```python
from build123d import *

# Parameters (mm, degrees)
F1_DEPTH     = 2
F2_W         = 44.2697719236
F2_H         = 2
F2_W_2       = 43.7677401211
F2_W_3       = 43.2657083186
F2_W_4       = 42.7408568887
F2_W_5       = 42.1931858314
F2_W_6       = 41.5998755193
F2_W_7       = 40.9609259524
F2_W_8       = 40.2763371308
F2_W_9       = 39.5461090544
F2_W_10      = 38.7702417233
F2_W_11      = 37.9487351373
F2_W_12      = 37.0815892966
F2_W_13      = 36.1688042011
F2_W_14      = 35.2103798508
F2_W_15      = 34.2063162458
F3_DEPTH     = 1
F4_T1_DEPTH  = 50.2158074986
F4_T3_DEPTH  = 3.0186569416
F4_T5_DEPTH  = 47.197150557
F4_T7_DEPTH  = 49.7137756961
F4_T9_DEPTH  = 49.2117438936
F4_T11_DEPTH = 48.6868924637
F4_T13_DEPTH = 48.1392214064
F4_T15_DEPTH = 47.5459110943
F4_T17_DEPTH = 46.9069615275
F4_T19_DEPTH = 46.2223727058
F4_T21_DEPTH = 45.4921446294
F4_T23_DEPTH = 44.7162772983
F4_T25_DEPTH = 43.8947707123
F4_T27_DEPTH = 43.0276248716
F4_T29_DEPTH = 42.1148397761
F4_T31_DEPTH = 41.1564154259
F4_T33_DEPTH = 40.1523518208


# Not quite as in the source:
# - a fillet or chamfer that OpenCascade refuses, or shapes differently, is made with other operations: its cross-section is extruded or revolved along the edge and cut away or added


with BuildPart() as f1:
    # F0 (on Top) → F1 (new body)
    with BuildSketch(Plane.XY):
        Polygon((17.9405650105, 218.366242675), (-15.0594349895, 218.366242675), (-21.0594349895, -44.5653073527), (23.9405650105, -44.5653073527), align=None)
    extrude(amount=F1_DEPTH)

    # F2 (on face) → F3 (join)
    with BuildSketch(Plane.XY.offset(2)):
        with Locations((1.4633846378, -28.5653073527)):
            Rectangle(F2_W, F2_H)
        with Locations((1.4405650105, -18.5653073527)):
            Rectangle(F2_W_2, F2_H)
        with Locations((1.4405650105, -7.5653073527)):
            Rectangle(F2_W_3, F2_H)
        with Locations((1.4405650105, 3.9346926473)):
            Rectangle(F2_W_4, F2_H)
        with Locations((1.4405650105, 15.9346926473)):
            Rectangle(F2_W_5, F2_H)
        with Locations((1.4405650105, 28.9346926473)):
            Rectangle(F2_W_6, F2_H)
        with Locations((1.4405650105, 42.9346926473)):
            Rectangle(F2_W_7, F2_H)
        with Locations((1.4405650105, 57.9346926473)):
            Rectangle(F2_W_8, F2_H)
        with Locations((1.4405650105, 73.9346926473)):
            Rectangle(F2_W_9, F2_H)
        with Locations((1.4405650105, 90.9346926473)):
            Rectangle(F2_W_10, F2_H)
        with Locations((1.4405650105, 108.9346926473)):
            Rectangle(F2_W_11, F2_H)
        with Locations((1.4405650105, 127.9346926473)):
            Rectangle(F2_W_12, F2_H)
        with Locations((1.4405650105, 147.9346926473)):
            Rectangle(F2_W_13, F2_H)
        with Locations((1.4405650105, 168.9346926473)):
            Rectangle(F2_W_14, F2_H)
        with Locations((1.4405650105, 190.9346926473)):
            Rectangle(F2_W_15, F2_H)
    extrude(amount=F3_DEPTH)

    # F4: fillet of radius 1.2071067812 on 30 edges, made by hand

    # F4_s2 → F4_t1 (cut)
    with BuildSketch(Plane.YZ.offset(-23.6445191115)):
        with BuildLine():
            ThreePointArc((-29.5653073527, 2), (-29.1529872247, 2.7167727513), (-28.3761002377, 3))
            Line((-28.3761002377, 3), (-29.5653073527, 3))
            Line((-29.5653073527, 3), (-29.5653073527, 2))
        make_face()
    extrude(amount=F4_T1_DEPTH, mode=Mode.SUBTRACT)

    # F4_s4 → F4_t3 (cut)
    with BuildSketch(Plane.YZ.offset(23.5526314455)):
        with BuildLine():
            ThreePointArc((-27.5653073527, 2), (-27.9776274807, 2.7167727513), (-28.7545144677, 3))
            Line((-28.7545144677, 3), (-27.5653073527, 3))
            Line((-27.5653073527, 3), (-27.5653073527, 2))
        make_face()
    extrude(amount=F4_T3_DEPTH, mode=Mode.SUBTRACT)

    # F4_s6 → F4_t5 (cut)
    with BuildSketch(Plane.YZ.offset(-23.6445191115)):
        with BuildLine():
            ThreePointArc((-27.5653073527, 2), (-27.9776274807, 2.7167727513), (-28.7545144677, 3))
            Line((-28.7545144677, 3), (-27.5653073527, 3))
            Line((-27.5653073527, 3), (-27.5653073527, 2))
        make_face()
    extrude(amount=F4_T5_DEPTH, mode=Mode.SUBTRACT)

    # F4_s8 → F4_t7 (cut)
    with BuildSketch(Plane.YZ.offset(-23.4163228376)):
        with BuildLine():
            ThreePointArc((-19.5653073527, 2), (-19.1529872247, 2.7167727513), (-18.3761002377, 3))
            Line((-18.3761002377, 3), (-19.5653073527, 3))
            Line((-19.5653073527, 3), (-19.5653073527, 2))
        make_face()
        with BuildLine():
            ThreePointArc((-17.5653073527, 2), (-17.9776274807, 2.7167727513), (-18.7545144677, 3))
            Line((-18.7545144677, 3), (-17.5653073527, 3))
            Line((-17.5653073527, 3), (-17.5653073527, 2))
        make_face()
    extrude(amount=F4_T7_DEPTH, mode=Mode.SUBTRACT)

    # F4_s10 → F4_t9 (cut)
    with BuildSketch(Plane.YZ.offset(-23.1653069363)):
        with BuildLine():
            ThreePointArc((-8.5653073527, 2), (-8.1529872247, 2.7167727513), (-7.3761002377, 3))
            Line((-7.3761002377, 3), (-8.5653073527, 3))
            Line((-8.5653073527, 3), (-8.5653073527, 2))
        make_face()
        with BuildLine():
            ThreePointArc((-6.5653073527, 2), (-6.9776274807, 2.7167727513), (-7.7545144677, 3))
            Line((-7.7545144677, 3), (-6.5653073527, 3))
            Line((-6.5653073527, 3), (-6.5653073527, 2))
        make_face()
    extrude(amount=F4_T9_DEPTH, mode=Mode.SUBTRACT)

    # F4_s12 → F4_t11 (cut)
    with BuildSketch(Plane.YZ.offset(-22.9028812214)):
        with BuildLine():
            ThreePointArc((2.9346926473, 2), (3.3470127753, 2.7167727513), (4.1238997623, 3))
            Line((4.1238997623, 3), (2.9346926473, 3))
            Line((2.9346926473, 3), (2.9346926473, 2))
        make_face()
        with BuildLine():
            ThreePointArc((4.9346926473, 2), (4.5223725193, 2.7167727513), (3.7454855323, 3))
            Line((3.7454855323, 3), (4.9346926473, 3))
            Line((4.9346926473, 3), (4.9346926473, 2))
        make_face()
    extrude(amount=F4_T11_DEPTH, mode=Mode.SUBTRACT)

    # F4_s14 → F4_t13 (cut)
    with BuildSketch(Plane.YZ.offset(-22.6290456927)):
        with BuildLine():
            ThreePointArc((14.9346926473, 2), (15.3470127753, 2.7167727513), (16.1238997623, 3))
            Line((16.1238997623, 3), (14.9346926473, 3))
            Line((14.9346926473, 3), (14.9346926473, 2))
        make_face()
        with BuildLine():
            ThreePointArc((16.9346926473, 2), (16.5223725193, 2.7167727513), (15.7454855323, 3))
            Line((15.7454855323, 3), (16.9346926473, 3))
            Line((16.9346926473, 3), (16.9346926473, 2))
        make_face()
    extrude(amount=F4_T13_DEPTH, mode=Mode.SUBTRACT)

    # F4_s16 → F4_t15 (cut)
    with BuildSketch(Plane.YZ.offset(-22.3323905367)):
        with BuildLine():
            ThreePointArc((27.9346926473, 2), (28.3470127753, 2.7167727513), (29.1238997623, 3))
            Line((29.1238997623, 3), (27.9346926473, 3))
            Line((27.9346926473, 3), (27.9346926473, 2))
        make_face()
        with BuildLine():
            ThreePointArc((29.9346926473, 2), (29.5223725193, 2.7167727513), (28.7454855323, 3))
            Line((28.7454855323, 3), (29.9346926473, 3))
            Line((29.9346926473, 3), (29.9346926473, 2))
        make_face()
    extrude(amount=F4_T15_DEPTH, mode=Mode.SUBTRACT)

    # F4_s18 → F4_t17 (cut)
    with BuildSketch(Plane.YZ.offset(-22.0129157533)):
        with BuildLine():
            ThreePointArc((41.9346926473, 2), (42.3470127753, 2.7167727513), (43.1238997623, 3))
            Line((43.1238997623, 3), (41.9346926473, 3))
            Line((41.9346926473, 3), (41.9346926473, 2))
        make_face()
        with BuildLine():
            ThreePointArc((43.9346926473, 2), (43.5223725193, 2.7167727513), (42.7454855323, 3))
            Line((42.7454855323, 3), (43.9346926473, 3))
            Line((43.9346926473, 3), (43.9346926473, 2))
        make_face()
    extrude(amount=F4_T17_DEPTH, mode=Mode.SUBTRACT)

    # F4_s20 → F4_t19 (cut)
    with BuildSketch(Plane.YZ.offset(-21.6706213425)):
        with BuildLine():
            ThreePointArc((56.9346926473, 2), (57.3470127753, 2.7167727513), (58.1238997623, 3))
            Line((58.1238997623, 3), (56.9346926473, 3))
            Line((56.9346926473, 3), (56.9346926473, 2))
        make_face()
        with BuildLine():
            ThreePointArc((58.9346926473, 2), (58.5223725193, 2.7167727513), (57.7454855323, 3))
            Line((57.7454855323, 3), (58.9346926473, 3))
            Line((58.9346926473, 3), (58.9346926473, 2))
        make_face()
    extrude(amount=F4_T19_DEPTH, mode=Mode.SUBTRACT)

    # F4_s22 → F4_t21 (cut)
    with BuildSketch(Plane.YZ.offset(-21.3055073043)):
        with BuildLine():
            ThreePointArc((72.9346926473, 2), (73.3470127753, 2.7167727513), (74.1238997623, 3))
            Line((74.1238997623, 3), (72.9346926473, 3))
            Line((72.9346926473, 3), (72.9346926473, 2))
        make_face()
        with BuildLine():
            ThreePointArc((74.9346926473, 2), (74.5223725193, 2.7167727513), (73.7454855323, 3))
            Line((73.7454855323, 3), (74.9346926473, 3))
            Line((74.9346926473, 3), (74.9346926473, 2))
        make_face()
    extrude(amount=F4_T21_DEPTH, mode=Mode.SUBTRACT)

    # F4_s24 → F4_t23 (cut)
    with BuildSketch(Plane.YZ.offset(-20.9175736387)):
        with BuildLine():
            ThreePointArc((89.9346926473, 2), (90.3470127753, 2.7167727513), (91.1238997623, 3))
            Line((91.1238997623, 3), (89.9346926473, 3))
            Line((89.9346926473, 3), (89.9346926473, 2))
        make_face()
        with BuildLine():
            ThreePointArc((91.9346926473, 2), (91.5223725193, 2.7167727513), (90.7454855323, 3))
            Line((90.7454855323, 3), (91.9346926473, 3))
            Line((91.9346926473, 3), (91.9346926473, 2))
        make_face()
    extrude(amount=F4_T23_DEPTH, mode=Mode.SUBTRACT)

    # F4_s26 → F4_t25 (cut)
    with BuildSketch(Plane.YZ.offset(-20.5068203457)):
        with BuildLine():
            ThreePointArc((107.9346926473, 2), (108.3470127753, 2.7167727513), (109.1238997623, 3))
            Line((109.1238997623, 3), (107.9346926473, 3))
            Line((107.9346926473, 3), (107.9346926473, 2))
        make_face()
        with BuildLine():
            ThreePointArc((109.9346926473, 2), (109.5223725193, 2.7167727513), (108.7454855323, 3))
            Line((108.7454855323, 3), (109.9346926473, 3))
            Line((109.9346926473, 3), (109.9346926473, 2))
        make_face()
    extrude(amount=F4_T25_DEPTH, mode=Mode.SUBTRACT)

    # F4_s28 → F4_t27 (cut)
    with BuildSketch(Plane.YZ.offset(-20.0732474254)):
        with BuildLine():
            ThreePointArc((126.9346926473, 2), (127.3470127753, 2.7167727513), (128.1238997623, 3))
            Line((128.1238997623, 3), (126.9346926473, 3))
            Line((126.9346926473, 3), (126.9346926473, 2))
        make_face()
        with BuildLine():
            ThreePointArc((128.9346926473, 2), (128.5223725193, 2.7167727513), (127.7454855323, 3))
            Line((127.7454855323, 3), (128.9346926473, 3))
            Line((128.9346926473, 3), (128.9346926473, 2))
        make_face()
    extrude(amount=F4_T27_DEPTH, mode=Mode.SUBTRACT)

    # F4_s30 → F4_t29 (cut)
    with BuildSketch(Plane.YZ.offset(-19.6168548776)):
        with BuildLine():
            ThreePointArc((146.9346926473, 2), (147.3470127753, 2.7167727513), (148.1238997623, 3))
            Line((148.1238997623, 3), (146.9346926473, 3))
            Line((146.9346926473, 3), (146.9346926473, 2))
        make_face()
        with BuildLine():
            ThreePointArc((148.9346926473, 2), (148.5223725193, 2.7167727513), (147.7454855323, 3))
            Line((147.7454855323, 3), (148.9346926473, 3))
            Line((148.9346926473, 3), (148.9346926473, 2))
        make_face()
    extrude(amount=F4_T29_DEPTH, mode=Mode.SUBTRACT)

    # F4_s32 → F4_t31 (cut)
    with BuildSketch(Plane.YZ.offset(-19.1376427025)):
        with BuildLine():
            ThreePointArc((167.9346926473, 2), (168.3470127753, 2.7167727513), (169.1238997623, 3))
            Line((169.1238997623, 3), (167.9346926473, 3))
            Line((167.9346926473, 3), (167.9346926473, 2))
        make_face()
        with BuildLine():
            ThreePointArc((169.9346926473, 2), (169.5223725193, 2.7167727513), (168.7454855323, 3))
            Line((168.7454855323, 3), (169.9346926473, 3))
            Line((169.9346926473, 3), (169.9346926473, 2))
        make_face()
    extrude(amount=F4_T31_DEPTH, mode=Mode.SUBTRACT)

    # F4_s34 → F4_t33 (cut)
    with BuildSketch(Plane.YZ.offset(-18.6356109)):
        with BuildLine():
            ThreePointArc((189.9346926473, 2), (190.3470127753, 2.7167727513), (191.1238997623, 3))
            Line((191.1238997623, 3), (189.9346926473, 3))
            Line((189.9346926473, 3), (189.9346926473, 2))
        make_face()
        with BuildLine():
            ThreePointArc((191.9346926473, 2), (191.5223725193, 2.7167727513), (190.7454855323, 3))
            Line((190.7454855323, 3), (191.9346926473, 3))
            Line((191.9346926473, 3), (191.9346926473, 2))
        make_face()
    extrude(amount=F4_T33_DEPTH, mode=Mode.SUBTRACT)


solid = f1.part
```
Source: CAD feature listing. Evaluate the final solid. Frame: model axes, mm. A direction names the side the tool comes from. Give positions to 0.01 mm unless a question says otherwise; leave off trailing zeros. Write each loop counter-clockwise with the first axis right and the second up, starting at its lowest first coordinate (ties: lowest second). Pieces come first, ordered by that corner, then holes. Notation, with made-up numbers: (-29.75, 39) - (-2.75, 39) arc R16 cw to (-2.75, 66) - close; hole circle Ø3 at (-6.75, 1). An arc over 180 degrees is marked (long way). One line per item, written item: value. Start each with the question number.
Q1. First-contact query: pin 1 Ø3 at (x, y) = (16, 18) entering from +Z; pin 2 Ø0.8 at (y, z) = (58, 2.5) entering from -X; pin 3 Ø5 at (x, y) = (13, 49) entering from +Z. Flat tips, straight axial feed; report the tip coordinate or a pass-through.
Q2. Material intervals for probe 1 along X at (y, z) = (29, 1.5); probe 2 along Z at (x, y) = (-7, 64); probe 3 along X at (y, z) = (-7, 0.8), sorted ascending. Write a range as from..to.
Q3. Set-up query: faces 3 (the face through (1, -36, 2)), 4 (the face through (1, -24, 2)), 5 (the face through (1, 89, 0)). Return all of +Z, -Z, +X, -X, +Y, -Y with unobstructed straight access to the full face (end or side cutting, diameter ignored); none if empty.
Q4. Section query A-A, the plane z = 0.8. Return the cut outline in (x, y).
Q5. Draft query along Y for faces 1 (the face through (1, 157, 2)), 2 (the face through (1, 205, 2)). Return one class per face: +Y half, -Y half, draft (parallel to the pull), parting line (faces both ways), or undercut.
Q6. Section query B-B, the plane y = 124.5. Return the cut outline in (x, z), then the cut area to 3 significant figures.
Answer:
1. pin 1: stops at z = 2.74
1. pin 2: stops at x = -18.7
1. pin 3: stops at z = 2
2. probe 1: x = -19.38..22.26
2. probe 2: z = 0..2
2. probe 3: x = -20.2..23.08
3. face 3: +Z, +X, -X, -Y
3. face 4: +Z, +X, -X
3. face 5: -Z, +X, -X, +Y, -Y
4. outline: (-21.06, -44.57) - (23.94, -44.57) - (17.94, 218.37) - (-15.06, 218.37) - close
5. face 1: undercut
5. face 2: draft
6. outline: (-17.2, 0) - (20.08, 0) - (20.08, 2) - (-17.2, 2) - close
6. area: 74.6 mm2
